The listing builds one solid part. Answer for the finished solid, in the listing's coordinates (mm). Face numbers are marked on the shaded views. Coordinates: 2 decimals unless noted, no trailing zeros. Order: outer loops, then holes, each group sorted by start corner. A loop starts at its lowest first (then second) coordinate and runs counter-clockwise, first axis right, second up. Notation, with made-up numbers: (79.5, 17.5) - (87.5, 17.5) arc R13 cw to (87.5, 24.5) - close; hole circle Ø11 at (54.25, 25.25). An arc over 180 degrees is marked (long way). Use a Markdown table: item, result. Add a question column.
Item 1: The mould has two halves that part along Z. Classify the marked faces 1, 2 and 3: released by +Z, released by -Z, zero draft, split by the parting line, or undercut.
Item 2: The part is cut by section C-C, the plane x = 8. Give the vertices of the cut face in (y, z).
Item 3: Flat-ended cylindrical pins translate along their axes: P1, Ø3, axis at y = -8, z = -8.5, coming from the +X side; P2, Ø3, axis at y = -9, z = 7, coming from the +X side; P3, Ø4, axis at x = 8, y = -10, coming from the -Z side. Find the tip coordinate at first contact, or state that the pin passes through.
Item 4: Find the intervals of material crossed by line 1 along Y through (x, z) = (4, 0); line 2 along Z through (x, y) = (1, 0.5); line 3 along Y through (x, z) = (9.5, 2.5), in increasing order.
Item 5: The part is cut by section A-A, the plane z = 0. Give the vertices of the cut face in (x, y).
from build123d import *

# Parameters (mm, degrees)
CHAMFER1_SIZE      = 1
FILLET1_R          = 1
SKETCH2_R          = 3.25
CUT_EXTRUDE1_DEPTH = 10


with BuildPart() as part:
    # Sketch1 → Revolve1 (revolve)
    with BuildSketch(Plane.XY, mode=Mode.PRIVATE) as revolve1_sk:
        Polygon((0, 7.5), (10, 7.5), (10, 10.5), (3, 10.5), (3, 13.5), (0, 13.5), align=None)
    revolve(revolve1_sk.sketch.rotate(Axis((0, 0, 0), (1, 0, 0)), 90), axis=Axis((0, 0, 0), (1, 0, 0)))

    # Chamfer1
    chamfer1_edges = [part.edges().sort_by_distance(p)[0] for p in [
        (0, 0, -13.5),
        (3, 0, -13.5),
        (10, 0, -10.5),
        (10, 0, -7.5),
        (0, 0, -7.5),
    ]]
    chamfer(chamfer1_edges, length=CHAMFER1_SIZE)

    # Fillet1
    fillet1_edges = [part.edges().sort_by_distance(p)[0] for p in [
        (3, 0, -10.5),
    ]]
    fillet(fillet1_edges, radius=FILLET1_R)

    # Sketch2 → Cut-Extrude1 (cut)
    with BuildSketch(Plane.ZY):
        with Locations((0, 14)):
            Circle(SKETCH2_R)
        with Locations((-14, 0)):
            Circle(SKETCH2_R)
        with Locations((0, -14)):
            Circle(SKETCH2_R)
        with Locations((14, 0)):
            Circle(SKETCH2_R)
    extrude(amount=-CUT_EXTRUDE1_DEPTH, mode=Mode.SUBTRACT)


solid = part.part
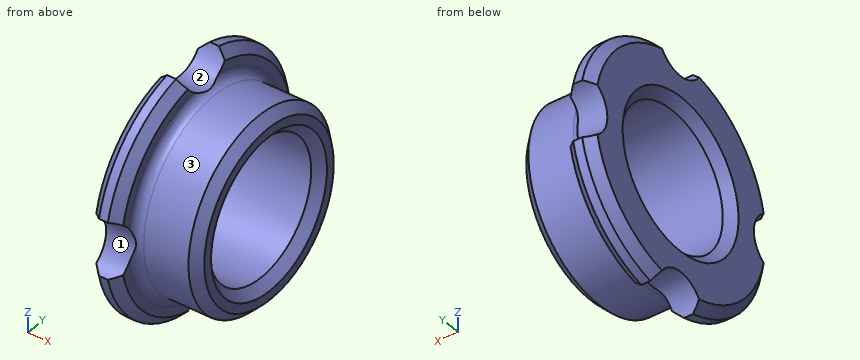
Solution:
| question | item | result |
|---|---|---|
| 1 | face 1 | undercut |
| 1 | face 2 | released by +Z |
| 1 | face 3 | split by the parting line |
| 2 | outline | circle Ø21 at (0, 0); hole circle Ø15 at (0, 0) |
| 3 | P1 | stops at x = 9.33 |
| 3 | P2 | stops at x = 9.6 |
| 3 | P3 | stops at z = -6.8 |
| 4 | line 1 | y = -10.5 to -7.5, 7.5 to 10.5 |
| 4 | line 2 | z = -10.79 to -7.48, 7.48 to 10.79 |
| 4 | line 3 | y = -9.68 to -7.6, 7.6 to 9.68 |
| 5 | outline | (0, -10.75) - (3.34, -10.75) arc R1 cw to (4, -10.5) - (9, -10.5) - (10, -9.5) - (10, -8.5) - (9, -7.5) - (1, -7.5) - (0, -8.5) - close; (0, 8.5) - (1, 7.5) - (9, 7.5) - (10, 8.5) - (10, 9.5) - (9, 10.5) - (4, 10.5) arc R1 cw to (3.34, 10.75) - (0, 10.75) - close |
